Work out the finished part from the listing and answer in its coordinate system (mm). Face numbers are marked on the shaded views. A direction names the side the tool comes from. Give positions to 0.01 mm unless a question says otherwise; leave off trailing zeros. Order: outer loops, then holes, each group sorted by start corner. A loop starts at its lowest first (then second) coordinate and runs counter-clockwise, first axis right, second up.
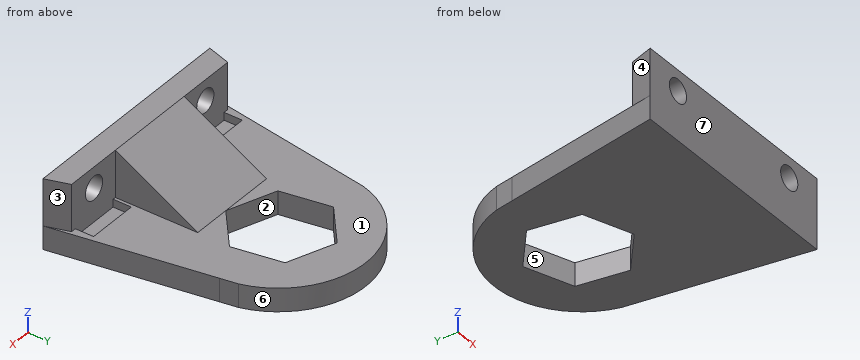
```python
from build123d import *

# Parameters (mm, degrees)
SKETCH_1_R          = 6.5
EXTRUDE_1_DEPTH     = 3
EXTRUDE_2_DEPTH     = 6
SKETCH_5_R          = 1.5
CUT_EXTRUDE_1_DEPTH = 6
EXTRUDE_3_DEPTH     = 3
SKETCH_7_R          = 7.581975651
EXTRUDE_4_DEPTH     = 3
CUT_EXTRUDE_2_DEPTH = 3
EXTRUDE_5_DEPTH     = 6
SKETCH_10_W         = 6.596302857
SKETCH_10_H         = 2.358868677
CUT_EXTRUDE_3_DEPTH = 1


with BuildPart() as part:
    # 草图1 → 凸台-拉伸1 (new body)
    with BuildSketch(Plane.XY):
        with BuildLine():
            Line((0, -11.15), (-14.569688113, -11.15))
            Line((-14.569688113, -11.15), (-10.110162273, 3.152379613))
            ThreePointArc((-10.110162273, 3.152379613), (0, 10.590225607), (10.110162273, 3.152379613))
            Line((10.110162273, 3.152379613), (14.569688113, -11.15))
            Line((14.569688113, -11.15), (0, -11.15))
        make_face()
        Circle(SKETCH_1_R, mode=Mode.SUBTRACT)
    extrude(amount=EXTRUDE_1_DEPTH)

    # 草图4 → 凸台-拉伸2 (add)
    with BuildSketch(Plane.XY.offset(3)):
        Polygon((0, -8.15), (13.63427891, -8.15), (14.569688113, -11.15), (-14.569688113, -11.15), (-13.63427891, -8.15), align=None)
    extrude(amount=EXTRUDE_2_DEPTH)

    # 草图5 → 切除-拉伸1 (cut)
    with BuildSketch(Plane(origin=(0, -8.15, 0), x_dir=(1, 0, 0), z_dir=(0, 1, 0))):
        with Locations(Location((-9.718639025, -6.319329225, 0), (0, 0, 270))):
            Circle(SKETCH_5_R)
        with Locations(Location((9.718639025, -6.319329225, 0), (0, 0, 180))):
            Circle(SKETCH_5_R)
    extrude(amount=-CUT_EXTRUDE_1_DEPTH, mode=Mode.SUBTRACT)

    # 草图6 → 凸台-拉伸3 (add)
    with BuildSketch(Plane(origin=(0, 0, 0), x_dir=(-1, 0, 0), z_dir=(0, 0, -1))):
        with BuildLine():
            Line((10.110162273, 3.152379613), (14.569688113, -11.15))
            Line((14.569688113, -11.15), (11.256321717, 9.136259589))
            Line((11.256321717, 9.136259589), (10.892618435, 11.363052016))
            ThreePointArc((10.892618435, 11.363052016), (0, 19.718638154), (-10.892618435, 11.363052016))
            Line((-10.892618435, 11.363052016), (-11.256321717, 9.136259589))
            Line((-11.256321717, 9.136259589), (-14.569688113, -11.15))
            Line((-14.569688113, -11.15), (-10.110162273, 3.152379613))
            ThreePointArc((-10.110162273, 3.152379613), (0, 10.590225607), (10.110162273, 3.152379613))
        make_face()
    extrude(amount=-EXTRUDE_3_DEPTH)

    # 草图7 → 凸台-拉伸4 (add)
    with BuildSketch(Plane(origin=(0, 0, 0), x_dir=(-1, 0, 0), z_dir=(0, 0, -1))):
        Circle(SKETCH_7_R)
    extrude(amount=-EXTRUDE_4_DEPTH)

    # 草图8 → 切除-拉伸2 (cut)
    with BuildSketch(Plane(origin=(0, 0, 0), x_dir=(-1, 0, 0), z_dir=(0, 0, -1))):
        Polygon((1.103523442, 15.221465243), (-4.966089039, 12.991411956), (-6.069612481, 6.619946712), (-1.103523442, 2.478534757), (4.966089039, 4.708588044), (6.069612481, 11.080053288), align=None)
    extrude(amount=-CUT_EXTRUDE_2_DEPTH, mode=Mode.SUBTRACT)

    # 草图9 → 凸台-拉伸5 (add, symmetric)
    with BuildSketch(Plane(origin=(0, 0, 0), x_dir=(0, 0, -1), z_dir=(1, 0, 0))):
        Polygon((-9, -8.15), (-3, 2.478534757), (-3, -8.15), align=None)
    extrude(amount=EXTRUDE_5_DEPTH, both=True)

    # 草图10 → 切除-拉伸3 (cut)
    with BuildSketch(Plane.XY.offset(3)):
        with Locations((-9.693347491, -6.970565662)):
            Rectangle(SKETCH_10_W, SKETCH_10_H)
        with Locations((9.693347491, -6.970565662)):
            Rectangle(SKETCH_10_W, SKETCH_10_H)
    extrude(amount=-CUT_EXTRUDE_3_DEPTH, mode=Mode.SUBTRACT)


solid = part.part
```
1. The part is cut by section B-B (y = 12). Write down the section's boundary in (x, z), then the cut area to 3 significant figures.
Findings below:
outline: (-10.7, 0) - (-4.97, 0) - (-4.97, 3) - (-10.7, 3) - close; (5.14, 0) - (10.7, 0) - (10.7, 3) - (5.14, 3) - close
area: 33.9 mm2
2. The part is cut by section C-C (z = 4.25). Write down the section's boundary in (x, y), then the cut area to 3 significant figures.
Findings below:
outline: (-14.57, -11.15) - (14.57, -11.15) - (13.63, -8.15) - (6, -8.15) - (6, 0.26) - (-6, 0.26) - (-6, -8.15) - (-13.63, -8.15) - close
area: 186 mm2
3. The mould has two halves that part along X. Classify the marked faces 4, 5, 6 and 7: pulls with the +X half, pulls with the -X half, needs draft (parallel to the pull), parting line crosses it, or undercut.
Findings below:
face 4: pulls with the -X half
face 5: undercut
face 6: parting line crosses it
face 7: needs draft
4. The part is cut by section D-D (x = -7.25). Write down the section's boundary in (y, z).
Findings below:
outline: (-11.15, 0) - (17.08, 0) - (17.08, 3) - (-5.79, 3) - (-5.79, 2) - (-8.15, 2) - (-8.15, 9) - (-11.15, 9) - close
5. Which of the six approach directions +Z, -Z, +X, -X, +Y, -Y give full straight-line access (tool end or side, diameter ignored) to the marked faces 1, 2 and 3?
Findings below:
face 1: +Z, +Y
face 2: +Z, -Z
face 3: +Z, +X, +Y
6. Given P1, Ø1.5, axis at x = -8, z = 7.5, coming from the +Y side; P2, Ø8.5, axis at x = 3, y = 6, coming from the +Z side; P3, Ø2.5, axis at x = -9.72, z = 6.32, coming from the -Y side; P4, Ø3, axis at y = 6, z = 3.5, coming from the -X side, each flat-ended and moving along its own axis, determine where each tip first touches the part or whether it passes through.
Findings below:
P1: stops at y = -8.15
P2: stops at z = 3.41
P3: passes through
P4: stops at x = -12
7. Straight lines are drawn through the part: probe 1 along X at (y, z) = (-10, 7.25); probe 2 along Z at (x, y) = (-6.5, 9); probe 3 along Y at (x, z) = (-0.75, 1.75). For each, find the intervals that lie inside material, in ascending order.
Findings below:
probe 1: x = -14.21 to -10.9, -8.54 to 8.54, 10.9 to 14.21
probe 2: z = 0 to 3
probe 3: y = -11.15 to 3.16, 15.09 to 19.69
8. The part is cut by section A-A (x = 2.5). Write down the section's boundary in (y, z).
Findings below:
outline: (-11.15, 0) - (3.64, 0) - (3.64, 3) - (2.48, 3) - (-8.15, 9) - (-11.15, 9) - close; (13.9, 0) - (19.44, 0) - (19.44, 3) - (13.9, 3) - close
